Could you check a few things on this model? Use its own coordinates, in mm. Face numbers are marked on the shaded views. A direction names the side the tool comes from. Give positions to 0.01 mm unless a question says otherwise; leave off trailing zeros. Loops run counter-clockwise (first coordinate to the right, second up) from the corner with the lowest first, then second, coordinate; pieces in that order, holes last. Notation, with made-up numbers: (3, 51) -> (17, 51) arc R21 ccw to (17, 57) -> close; hole circle Ø8 at (28, -33.5). An arc over 180 degrees is marked (long way). Write item = value, one per line. Start each with the question number.
1) I'm going to push flat-ended pins straight in: pin 1 Ø9 at (x, y) = (6, 4) entering from +Z; pin 2 Ø3 at (x, y) = (-34, -39.5) entering from +Z; pin 3 Ø10 at (x, z) = (-1.5, 37.5) entering from -Y. Where does each tip first touch, or does it pass through?
2) I want a section at B-B (z = 20). List the corners of the cut face in (x, y) for me, and give its area (3 significant figures).
3) I want a section at C-C (y = 38). List the corners of the cut face in (x, z) for me, and give its area (3 significant figures).
4) On a 3-axis mill with a long thin cutter (end or side, diameter ignored), from which of +Z, -Z, +X, -X, +Y, -Y can I reach the whole of each face in a straight line? I mean the marked faces 1 and 2. Say none if no direction works.
5) I want a section at D-D (z = 47.5). List the corners of the cut face in (x, y) for me, and give its area (3 significant figures).
6) I need wall thicknesses on probe 1 along Y at (x, z) = (0, 47); probe 2 along Y at (x, z) = (0.5, -8.5); probe 3 along X at (y, z) = (0, -3). Which ranges of each line are inside material? Lowest first, please. Write a range as from..to.
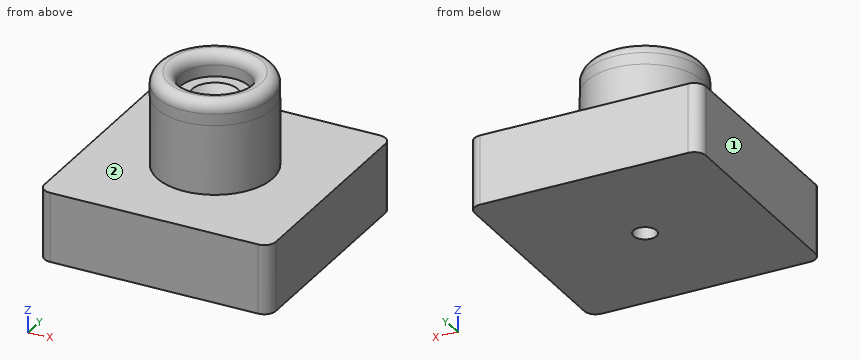
from build123d import *

# Parameters (mm, degrees)
F1_DEPTH       = 50
F0_W           = 25
F0_H           = 30
F4_D           = 10
F4_CSINK_D     = 20
F4_CSINK_ANGLE = 90
F5_R           = 5
F3_R           = 25
F3_R_2         = 15
F6_DEPTH       = 10
F7_R           = 4.99999


# Not quite as in the source:
# - a fillet or chamfer is up to 0.001 mm smaller than in the source, because OpenCascade refuses the exact size


with BuildPart() as f1:
    # F0 (on Front) → F1 (new body, symmetric)
    with BuildSketch(Plane.XZ):
        Polygon((50, 15), (25, 15), (0, 15), (0, -15), (50, -15), align=None)
        Polygon((0, -15), (0, 15), (-25, 15), (-50, 15), (-50, -15), align=None)
    extrude(amount=F1_DEPTH, both=True)

    # F0 (on Front) → F2 (revolve)
    with BuildSketch(Plane.XZ):
        with Locations((-12.5, 30)):
            Rectangle(F0_W, F0_H)
    revolve(axis=Axis((0, 0, 15), (0, 0, -1)))

    # F4 (through all)
    with Locations(Plane.XY.offset(45)):
        with Locations((0, 0)):
            CounterSinkHole(F4_D / 2, F4_CSINK_D / 2, counter_sink_angle=F4_CSINK_ANGLE)

    # F5
    f5_edges = [f1.edges().sort_by_distance(p)[0] for p in [
        (-50, 50, 0),
        (50, 50, 0),
        (50, -50, 0),
        (-50, -50, 0),
    ]]
    fillet(f5_edges, radius=F5_R)

    # F3 (on face) → F6 (join)
    with BuildSketch(Plane.XY.offset(45)):
        Circle(F3_R)
        Circle(F3_R_2, mode=Mode.SUBTRACT)
    extrude(amount=F6_DEPTH)

    # F7 (radius 5 in the source; OpenCascade refuses exactly that, so slightly less here)
    f7_edges = [f1.edges().sort_by_distance(p)[0] for p in [
        (-25, 0, 55),
        (-25, 0, 30),
        (-15, 0, 55),
    ]]
    fillet(f7_edges, radius=F7_R)


solid = f1.part
Answer list:
q1.pin_1 = 45
q1.pin_2 = 15
q1.pin_3 = -25
q2.outline = circle Ø50 at (0, 0); hole circle Ø10 at (0, 0)
q2.area = 1,880 mm^2
q3.outline = (-50, -15) -> (50, -15) -> (50, 15) -> (-50, 15) -> close
q3.area = 3,000 mm^2
q4.face_1 = +Z, -Z, -X, +Y, -Y
q4.face_2 = +Z
q5.outline = circle Ø50 at (0, 0); hole circle Ø30 at (0, 0)
q5.area = 1,260 mm^2
q6.probe_1 = -25..-15, 15..25
q6.probe_2 = -50..-4.97, 4.97..50
q6.probe_3 = -50..-5, 5..50
